Part model, mm, in its own coordinate system. A direction names the side the tool comes from. Round coordinates to 2 decimals unless told otherwise and drop trailing zeros. Loops run counter-clockwise (first coordinate to the right, second up) from the corner with the lowest first, then second, coordinate; pieces in that order, holes last.
1) Mould opens along X. For faces 4 (the flat face through (6.6, -11, 13)), 5 (the cylindrical face through (32.85, 7.78, -3.77)), 6 (the conical face through (32.59, 12.21, -2.38)), 7 (the flat face through (15, 10, 45)) say: +X half, -X half, draft (parallel to the pull), parting line (faces both ways), or undercut.
2) Band-saw the part on A-A, the plane x = 34. Write the cut outline in (y, z), then the cut area to 3 significant figures.
3) Drop flat-ended pins along their axis: P1, Ø4.5, axis at x = -1, y = 11, coming from the +Z side; P2, Ø2, axis at x = 26, z = 39, coming from the +Y side; P3, Ø7.5, axis at y = 7, z = 32, coming from the +X side; P4, Ø12, axis at x = 13.5, z = 38, coming from the -Y side. Give the stop position or say it passes through.
4) 3-axis set-ups, long thin cutter, end or side, ignore diameter. For faces 1 (the flat face through (6, 10, 25)), 2 (the flat face through (6.6, 10, 34)), 3 (the flat face through (15, 1.6, 34)): which of +Z, -Z, +X, -X, +Y, -Y reach the whole face in a straight line?
5) Probe line 1 (X direction, y = 10, z = -3); line 2 (Z direction, x = 5.5, y = 6); line 3 (Y direction, x = 16.5, z = 1). List the from-to ranges inside material, lowest first.
6) Band-saw the part on D-D, the plane x = 20.5. Write the cut outline in (y, z).
7) Band-saw the part on B-B, the plane y = -10.5. Write the cut outline in (x, z).
8) Band-saw the part on C-C, the plane z = 14. Write the cut outline in (x, y), then the cut area to 3 significant figures.
from build123d import *

# Parameters (mm, degrees)
F0_W            = 20
F0_H            = 20
F1_DEPTH        = 25
F0_W_2          = 5
F2_DEPTH        = 5
F3_W            = 16.8
F3_H            = 16.8
F4_DEPTH        = 20
F5_W            = 20
F5_H            = 20
F6_DEPTH        = 2
F7_SIZE         = 1
F8_W            = 16.8
F8_H            = 16.8
F9_DEPTH        = 20
F10_SIZE        = 1
F11_D           = 5
F11_CSINK_D     = 10
F11_CSINK_ANGLE = 90


with BuildPart() as f1:
    # F0 (on Top) → F1 (new body)
    with BuildSketch(Plane.XY):
        with Locations((15, 10)):
            Rectangle(F0_W, F0_H)
    extrude(amount=F1_DEPTH)

    # F0 (on Top) → F2 (join)
    with BuildSketch(Plane.XY):
        with Locations((2.5, 10)):
            Rectangle(F0_W_2, F0_H)
        with BuildLine():
            ThreePointArc((0, 20), (-10, 10), (0, 0))
            Line((0, 0), (0, 20))
        make_face()
        with Locations((15, 10)):
            Rectangle(F0_W, F0_H)
        with Locations((27.5, 10)):
            Rectangle(F0_W_2, F0_H)
        with BuildLine():
            Line((30, 20), (30, 0))
            ThreePointArc((30, 0), (40, 10), (30, 20))
        make_face()
    extrude(amount=-F2_DEPTH)

    # F3 (on face) → F4 (join)
    with BuildSketch(Plane.XY.offset(25)):
        with Locations((15, 10)):
            Rectangle(F3_W, F3_H)
    extrude(amount=F4_DEPTH)

    # F5 (on face) → F6 (join)
    with BuildSketch(Plane.XZ):
        with Locations((15, 13)):
            Rectangle(F5_W, F5_H)
    extrude(amount=F6_DEPTH)

    # F7
    f7_edges = [f1.edges().sort_by_distance(p)[0] for p in [
        (23.4, 18.4, 35),
        (6.6, 18.4, 35),
        (15, 18.4, 45),
        (6.6, 10, 45),
        (23.4, 10, 45),
        (15, 1.6, 45),
        (23.4, 1.6, 35),
        (6.6, 1.6, 35),
    ]]
    chamfer(f7_edges, length=F7_SIZE)

    # F8 (on face) → F9 (join)
    with BuildSketch(Plane.XZ.offset(2)):
        with Locations((15, 13)):
            Rectangle(F8_W, F8_H)
    extrude(amount=F9_DEPTH)

    # F10
    f10_edges = [f1.edges().sort_by_distance(p)[0] for p in [
        (23.4, -12, 21.4),
        (15, -22, 21.4),
        (6.6, -12, 21.4),
        (23.4, -22, 13),
        (23.4, -12, 4.6),
        (6.6, -12, 4.6),
        (6.6, -22, 13),
        (15, -22, 4.6),
    ]]
    chamfer(f10_edges, length=F10_SIZE)

    # F11 (through all)
    with Locations(Plane.XY):
        with Locations((-4, 10), (34, 10)):
            CounterSinkHole(F11_D / 2, F11_CSINK_D / 2, counter_sink_angle=F11_CSINK_ANGLE)


solid = f1.part
Reported:
1. face 4: -X half
1. face 5: undercut
1. face 6: undercut
1. face 7: draft
2. outline: (0.83, -5) - (7.5, -5) - (7.5, -2.5) - (5, 0) - (0.83, 0) - close; (12.5, -5) - (19.17, -5) - (19.17, 0) - (15, 0) - (12.5, -2.5) - close
2. area: 60.4 mm2
3. P1: stops at z = 0
3. P2: passes through
3. P3: stops at x = 23.4
3. P4: stops at y = 1.6
4. face 1: +Z
4. face 2: +Z, -X, +Y, -Y
4. face 3: +Z, +X, -X, -Y
5. line 1: x = -10 to -6.5, -1.5 to 31.5, 36.5 to 40
5. line 2: z = -5 to 25
5. line 3: y = 0 to 20
6. outline: (-22, 5.6) - (-21, 4.6) - (-2, 4.6) - (-2, 3) - (0, 3) - (0, -5) - (20, -5) - (20, 25) - (18.4, 25) - (18.4, 44) - (17.4, 45) - (2.6, 45) - (1.6, 44) - (1.6, 25) - (0, 25) - (0, 23) - (-2, 23) - (-2, 21.4) - (-21, 21.4) - (-22, 20.4) - close
7. outline: (6.6, 5.6) - (7.6, 4.6) - (22.4, 4.6) - (23.4, 5.6) - (23.4, 20.4) - (22.4, 21.4) - (7.6, 21.4) - (6.6, 20.4) - close
8. outline: (5, -2) - (6.6, -2) - (6.6, -21) - (7.6, -22) - (22.4, -22) - (23.4, -21) - (23.4, -2) - (25, -2) - (25, 20) - (5, 20) - close
8. area: 775 mm2
